```python
from build123d import *

# Parameters (mm, degrees)
SKETCH1_R           = 13.5
BOSS_EXTRUDE1_DEPTH = 32
BOSS_EXTRUDE2_DEPTH = 24


with BuildPart() as part:
    # Sketch1 → Boss-Extrude1 (new body)
    with BuildSketch(Plane.XY):
        Circle(SKETCH1_R)
    extrude(amount=BOSS_EXTRUDE1_DEPTH)

    # Sketch2 → Boss-Extrude2 (add)
    with BuildSketch(Plane.XY.offset(32)):
        with BuildLine():
            Line((-2.75, -3.75), (2.75, -3.75))
            ThreePointArc((2.75, -3.75), (3.457106781, -3.457106781), (3.75, -2.75))
            Line((3.75, -2.75), (3.75, 2.75))
            ThreePointArc((3.75, 2.75), (3.457106781, 3.457106781), (2.75, 3.75))
            Line((2.75, 3.75), (-2.75, 3.75))
            ThreePointArc((-2.75, 3.75), (-3.457106781, 3.457106781), (-3.75, 2.75))
            Line((-3.75, 2.75), (-3.75, -2.75))
            ThreePointArc((-3.75, -2.75), (-3.457106781, -3.457106781), (-2.75, -3.75))
        make_face()
    extrude(amount=BOSS_EXTRUDE2_DEPTH)


solid = part.part
```
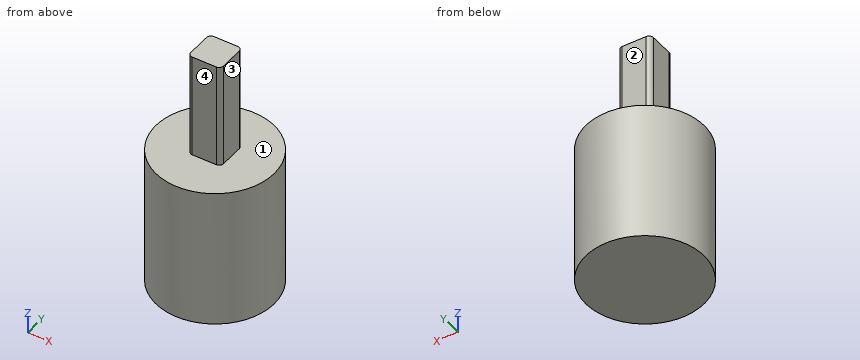
Geometry: final body of the model. Coordinates: model frame, mm. Face numbers are marked on the shaded views. A direction names the side the tool comes from. Coordinates: 2 decimals unless noted, no trailing zeros. Order: outer loops, then holes, each group sorted by start corner. A loop starts at its lowest first (then second) coordinate and runs counter-clockwise, first axis right, second up. Notation, with made-up numbers: M 55.5,10.5 L 90.5,10.5 A36 ccw 90.5,47.5 Z; hole C -6.5,69 d11. An arc over 180 degrees is marked long. Answer in a Markdown table with one row per item. Add a question column.
Q1. Section query B-B on z = 34. Return the cut outline in (x, y), and give its area (3 significant figures).
Q2. Section query A-A on y = 0. Return the cut outline in (x, z).
Q3. Reachability of the marked faces 1, 2, 3 and 4 from +Z, -Z, +X, -X, +Y, -Y: full face, straight path, thin tool, end or side. Return the list, or none.
Q4. Line query: L1, parallel to Z at x = 12, y = 1.5; L2, parallel to Y at x = -0.25, z = 33; L3, parallel to Y at x = -6.5, z = 2.5. Output: solid intervals per line, ascending.
Q5. Contact query for flat-ended pins moving along their axis: P1, Ø6, axis at x = -3.5, z = 22, coming from the +Y side; P2, Ø2, axis at x = 10.5, y = -7.5, coming from the +Z side; P3, Ø5, axis at x = -6, z = 15.5, coming from the -Y side. Output: stop coordinate, or through.
Q6. Section query D-D on z = 27. Return the cut outline in (x, y), and give its area (3 significant figures).
Q7. Section query C-C on x = -6. Return the cut outline in (y, z), and give its area (3 significant figures).
Completed:
| question | item | result |
|---|---|---|
| 1 | outline | M -3.75,-2.75 A1 ccw -2.75,-3.75 L 2.75,-3.75 A1 ccw 3.75,-2.75 L 3.75,2.75 A1 ccw 2.75,3.75 L -2.75,3.75 A1 ccw -3.75,2.75 Z |
| 1 | area | 55.4 mm2 |
| 2 | outline | M -13.5,0 L 13.5,0 L 13.5,32 L 3.75,32 L 3.75,56 L -3.75,56 L -3.75,32 L -13.5,32 Z |
| 3 | face 1 | +Z |
| 3 | face 2 | +Z, +X, -X, +Y |
| 3 | face 3 | +Z, +X, +Y, -Y |
| 3 | face 4 | +Z, +X, -X, -Y |
| 4 | L1 | z = 0 to 32 |
| 4 | L2 | y = -3.75 to 3.75 |
| 4 | L3 | y = -11.83 to 11.83 |
| 5 | P1 | stops at y = 13.49 |
| 5 | P2 | stops at z = 32 |
| 5 | P3 | stops at y = -13.04 |
| 6 | outline | C 0,0 d27 |
| 6 | area | 573 mm2 |
| 7 | outline | M -12.09,0 L 12.09,0 L 12.09,32 L -12.09,32 Z |
| 7 | area | 774 mm2 |
